from build123d import *

# Parameters (mm, degrees)
SKETCH1_W                               = 300
SKETCH1_H                               = 150
BOSS_EXTRUDE1_DEPTH                     = 22
CUT_EXTRUDE2_START                      = 22
SKETCH2_R                               = 36
CUT_EXTRUDE2_DEPTH                      = 19
SKETCH4_R                               = 18.5
CUT_EXTRUDE4_DEPTH                      = 3
CBORE_FOR_M8_HEX_HEAD_BOLT1_D           = 9
CBORE_FOR_M8_HEX_HEAD_BOLT1_CBORE_D     = 18.011
CBORE_FOR_M8_HEX_HEAD_BOLT1_CBORE_DEPTH = 5.3
TAP_DRILL_FOR_M6_TAP1_D                 = 5
CIRPATTERN1_COUNT                       = 4
MIRROR2_COPY_1_D                        = 5
MIRROR2_COPY_2_D                        = 5
MIRROR2_COPY_3_D                        = 5


with BuildPart() as part:
    # Sketch1 → Boss-Extrude1 (new body)
    with BuildSketch(Plane.XY):
        Rectangle(SKETCH1_W, SKETCH1_H)
    extrude(amount=BOSS_EXTRUDE1_DEPTH)

    # Sketch2 → Cut-Extrude2 (cut)
    with BuildSketch(Plane.XY.offset(CUT_EXTRUDE2_START)):
        with Locations((-60, 0)):
            Circle(SKETCH2_R)
    cut_extrude2 = extrude(amount=-CUT_EXTRUDE2_DEPTH, mode=Mode.SUBTRACT)

    # Sketch4 → Cut-Extrude4 (cut)
    with BuildSketch(Plane.XY):
        with Locations((-60, 0)):
            Circle(SKETCH4_R)
    cut_extrude4 = extrude(amount=CUT_EXTRUDE4_DEPTH, mode=Mode.SUBTRACT)

    # CBORE for M8 Hex Head Bolt1 (through all)
    with Locations(Plane(origin=(-140, 60, 22), x_dir=(1, 0, 0), z_dir=(0, 0, 1))):
        with Locations((0, 0), (0, -60), (0, -120)):
            cbore_for_m8_hex_head_bolt1 = CounterBoreHole(CBORE_FOR_M8_HEX_HEAD_BOLT1_D / 2, CBORE_FOR_M8_HEX_HEAD_BOLT1_CBORE_D / 2, CBORE_FOR_M8_HEX_HEAD_BOLT1_CBORE_DEPTH)

    # Mirror1: Cut-Extrude2, Cut-Extrude4, CBORE for M8 Hex Head Bolt1 across plane
    add(cut_extrude2.mirror(Plane(origin=(0, 0, 0), x_dir=(0, 0, 1), z_dir=(1, 0, 0))), mode=Mode.SUBTRACT)
    add(cut_extrude4.mirror(Plane(origin=(0, 0, 0), x_dir=(0, 0, 1), z_dir=(1, 0, 0))), mode=Mode.SUBTRACT)
    add(cbore_for_m8_hex_head_bolt1.mirror(Plane(origin=(0, 0, 0), x_dir=(0, 0, 1), z_dir=(1, 0, 0))), mode=Mode.SUBTRACT)

    # Tap Drill for M6 Tap1 (through all)
    with Locations(Plane(origin=(-29.9479618, 30.0520382, 22), x_dir=(1, 0, 0), z_dir=(0, 0, 1))):
        with Locations((0, 0)):
            tap_drill_for_m6_tap1 = Hole(TAP_DRILL_FOR_M6_TAP1_D / 2)

    # CirPattern1: Tap Drill for M6 Tap1 ×4 about axis
    cirpattern1_axis = Axis((-60, 0, 0), (0, 0, 1))
    for i in range(1, CIRPATTERN1_COUNT):
        add(tap_drill_for_m6_tap1.rotate(cirpattern1_axis, i * 360 / CIRPATTERN1_COUNT), mode=Mode.SUBTRACT)

    # Mirror2: Tap Drill for M6 Tap1 across plane
    add(tap_drill_for_m6_tap1.mirror(Plane(origin=(0, 0, 0), x_dir=(0, 0, 1), z_dir=(1, 0, 0))), mode=Mode.SUBTRACT)

    # Mirror2 copy 1 (through all)
    with Locations(Plane(origin=(90.0520382, 30.0520382, 22), x_dir=(0, 1, 0), z_dir=(0, 0, 1))):
        with Locations((0, 0)):
            Hole(MIRROR2_COPY_1_D / 2)

    # Mirror2 copy 2 (through all)
    with Locations(Plane(origin=(90.0520382, -30.0520382, 22), x_dir=(1, 0, 0), z_dir=(0, 0, 1))):
        with Locations((0, 0)):
            Hole(MIRROR2_COPY_2_D / 2)

    # Mirror2 copy 3 (through all)
    with Locations(Plane(origin=(29.9479618, -30.0520382, 22), x_dir=(0, -1, 0), z_dir=(0, 0, 1))):
        with Locations((0, 0)):
            Hole(MIRROR2_COPY_3_D / 2)


solid = part.part
Model file for the job. Use its own axes, mm. A direction names the side the tool comes from. Give positions to 0.01 mm unless a question says otherwise; leave off trailing zeros. Write each loop counter-clockwise with the first axis right and the second up, starting at its lowest first coordinate (ties: lowest second). Pieces come first, ordered by that corner, then holes. Notation, with made-up numbers: (-28, 80) -> (-7, 80) arc R17 ccw to (-7, 90) -> close; hole circle Ø2 at (18.5, -3). An arc over 180 degrees is marked (long way). Write item = value, one per line.
(1) Flat gauge pins, fed straight in: P1, Ø3, axis at x = -90.05, y = -30.05, coming from the -Z side (1 decimal); P2, Ø9, axis at x = 141, y = 56, coming from the +Z side. Where does each tip first touch, or does it go through?
Determined:
P1 = through
P2 = 16.7
(2) Slice it at C-C, the plane y = -60. Give the cut face in (x, z), then the cut area to 3 significant figures.
Determined:
outline = (-150, 0) -> (-144.5, 0) -> (-144.5, 16.7) -> (-149.01, 16.7) -> (-149.01, 22) -> (-150, 22) -> close; (-135.5, 0) -> (135.5, 0) -> (135.5, 16.7) -> (130.99, 16.7) -> (130.99, 22) -> (-130.99, 22) -> (-130.99, 16.7) -> (-135.5, 16.7) -> close; (144.5, 0) -> (150, 0) -> (150, 22) -> (149.01, 22) -> (149.01, 16.7) -> (144.5, 16.7) -> close
area = 6,110 mm2
(3) Probe line 1 along Y through (x, z) = (140, 10); line 2 along Y through (x, z) = (140, 19.25); line 3 along X through (y, z) = (-14.5, 16.25). List the from-to ranges inside material, lowest first.
Determined:
line_1 = -75 to -64.5, -55.5 to -4.5, 4.5 to 55.5, 64.5 to 75
line_2 = -75 to -69.01, -50.99 to -9.01, 9.01 to 50.99, 69.01 to 75
line_3 = -150 to -92.95, -27.05 to 27.05, 92.95 to 150
(4) Tool access for faces 1 (the face through (-2, -75, 11)), 2 (the face through (-148.997, 60.396, 19.387)): list every direction of +Z, -Z, +X, -X, +Y, -Y with a clear straight run to the whole face (end or side of a thin tool).
Determined:
face_1 = +Z, -Z, +X, -X, -Y
face_2 = +Z
(5) Slice it at B-B, the plane x = -140. Give the cut face in (y, z), then the cut area to 3 significant figures.
Determined:
outline = (-75, 0) -> (-64.5, 0) -> (-64.5, 16.7) -> (-69.01, 16.7) -> (-69.01, 22) -> (-75, 22) -> close; (-55.5, 0) -> (-4.5, 0) -> (-4.5, 16.7) -> (-9.01, 16.7) -> (-9.01, 22) -> (-50.99, 22) -> (-50.99, 16.7) -> (-55.5, 16.7) -> close; (4.5, 0) -> (55.5, 0) -> (55.5, 16.7) -> (50.99, 16.7) -> (50.99, 22) -> (9.01, 22) -> (9.01, 16.7) -> (4.5, 16.7) -> close; (64.5, 0) -> (75, 0) -> (75, 22) -> (69.01, 22) -> (69.01, 16.7) -> (64.5, 16.7) -> close
area = 2,560 mm2
(6) Slice it at A-A, the plane x = -60. Give the cut face in (y, z), then the cut area to 3 significant figures.
Determined:
outline = (-75, 0) -> (-18.5, 0) -> (-18.5, 3) -> (-36, 3) -> (-36, 22) -> (-75, 22) -> close; (18.5, 0) -> (75, 0) -> (75, 22) -> (36, 22) -> (36, 3) -> (18.5, 3) -> close
area = 1,820 mm2
(7) Mould opens along X. For faces 3 (the face through (150, -1, 11)), 4 (the face through (-150, -1, 11)), 5 (the face through (144.16, -1.72, 8.23)), 6 (the face through (-2, 75, 11)) say: released by +X, released by -X, zero draft, split by the parting line, or undercut.
Determined:
face_3 = released by +X
face_4 = released by -X
face_5 = undercut
face_6 = zero draft
(8) Slice it at D-D, the plane z = 8.5. Give the number of separate pieces and of enclosed holes in the cut face, then the cut area to 3 significant figures.
Determined:
separate_pieces = 1
enclosed_holes = 16
area = 36,300 mm2
